Model file for the job. Use its own axes, mm. Coordinates: 2 decimals unless noted, no trailing zeros. Write each loop counter-clockwise with the first axis right and the second up, starting at its lowest first coordinate (ties: lowest second). Pieces come first, ordered by that corner, then holes. Notation, with made-up numbers: M 46.25,59 L 87.25,59 A12 ccw 87.25,82 Z; hole C 2.25,7.5 d1. An arc over 180 degrees is marked long. Use CSV: the item, a comma, the result in double quotes. Start each with the question number.
from build123d import *

# Parameters (mm, degrees)
SKETCH_1_R      = 1.6
SKETCH_1_R_2    = 1.65
EXTRUDE_1_DEPTH = 3.5


with BuildPart() as part:
    # 草图1 → 凸台-拉伸1 (new body)
    with BuildSketch(Plane(origin=(0, 0, 0), x_dir=(1, 0, 0), z_dir=(0, 1, 0))):
        with BuildLine():
            Line((8304.199636281, 3083.866766782), (8349.87122342, 3094.435360284))
            ThreePointArc((8349.87122342, 3094.435360284), (8352.100502408, 3095.843120102), (8352.969436472, 3098.332382262))
            Line((8352.969436472, 3098.332382262), (8352.969436472, 3114.411583007))
            ThreePointArc((8352.969436472, 3114.411583007), (8352.5356662, 3116.223213635), (8351.328433707, 3117.641928507))
            Line((8351.328433707, 3117.641928507), (8305.656846567, 3150.99413426))
            ThreePointArc((8305.656846567, 3150.99413426), (8302.988857908, 3151.75183644), (8300.469422208, 3150.592215885))
            Line((8300.469422208, 3150.592215885), (8292.469422208, 3142.592215885))
            ThreePointArc((8292.469422208, 3142.592215885), (8291.496370678, 3141.008280638), (8291.344362542, 3139.155560023))
            Line((8291.344362542, 3139.155560023), (8299.344362542, 3087.155560023))
            ThreePointArc((8299.344362542, 3087.155560023), (8301.054579793, 3084.452030652), (8304.199636281, 3083.866766782))
        make_face()
        with Locations(Location((8348.969436472, 3098.332382262, 0), (0, 0, 270))):
            Circle(SKETCH_1_R, mode=Mode.SUBTRACT)
        with Locations(Location((8348.969436472, 3114.411583007, 0), (0, 0, 270))):
            Circle(SKETCH_1_R, mode=Mode.SUBTRACT)
        with Locations(Location((8303.297849333, 3131.76378876, 0), (0, 0, 270))):
            Circle(SKETCH_1_R, mode=Mode.SUBTRACT)
        with Locations(Location((8303.297849333, 3087.76378876, 0), (0, 0, 270))):
            Circle(SKETCH_1_R, mode=Mode.SUBTRACT)
        with Locations(Location((8303.297849333, 3147.76378876, 0), (0, 0, 270))):
            Circle(SKETCH_1_R_2, mode=Mode.SUBTRACT)
        with Locations(Location((8295.297849333, 3139.76378876, 0), (0, 0, 270))):
            Circle(SKETCH_1_R_2, mode=Mode.SUBTRACT)
        with Locations(Location((8311.297849333, 3139.76378876, 0), (0, 0, 270))):
            Circle(SKETCH_1_R_2, mode=Mode.SUBTRACT)
    extrude(amount=EXTRUDE_1_DEPTH)


solid = part.part
1) Wall check: L1, parallel to X at y = 2.25, z = -3132.5; L2, parallel to Z at x = 8349, y = 0.3; L3, parallel to X at y = 1.5, z = -3118.5. Give the ranges that are in metal, low to high. Write a range as [from, to].
2) Band-saw the part on C-C on z = -3123. List the corners of the cut face in (x, y).
3) Two-plate mould, pull along Z, no slides. Class faces 1 (the face through (8296.69, 1.73, -3138.88)), 2 (the face through (8352.548, 1.726, -3116.2)), 3 (the face through (8322, 3.5, -3111)): pulls with the +Z half, pulls with the -Z half, needs draft (parallel to the pull), parting line crosses it, or undercut.
4) Band-saw the part on A-A on y = 1.9. List the corners of the cut face in (x, z), then the cut area to 3 significant figures.
5) Band-saw the part on B-B on x = 8326. List the corners of the cut face in (y, z), then the cut area to 3 significant figures.
Findings below:
1,L1,"x = [8292.37, 8301.88], [8304.72, 8330.98]"
1,L2,"z = [-3119.34, -3116.01], [-3112.81, -3099.93], [-3096.73, -3094.23]"
1,L3,"x = [8294.52, 8350.15]"
2,outline,"M 8293.83,0 L 8343.99,0 L 8343.99,3.5 L 8293.83,3.5 Z"
3,face 1,"undercut"
3,face 2,"pulls with the -Z half"
3,face 3,"needs draft"
4,outline,"M 8291.34,-3139.16 A4 ccw 8292.47,-3142.59 L 8300.47,-3150.59 A4 ccw 8305.66,-3150.99 L 8351.33,-3117.64 A4 ccw 8352.97,-3114.41 L 8352.97,-3098.33 A4 ccw 8349.87,-3094.44 L 8304.2,-3083.87 A4 ccw 8299.34,-3087.16 Z; hole C 8295.3,-3139.76 d3.3; hole C 8303.3,-3147.76 d3.3; hole C 8303.3,-3131.76 d3.2; hole C 8303.3,-3087.76 d3.2; hole C 8311.3,-3139.76 d3.3; hole C 8348.97,-3114.41 d3.2; hole C 8348.97,-3098.33 d3.2"
4,area,"2,700 mm2"
5,outline,"M 0,-3136.14 L 3.5,-3136.14 L 3.5,-3088.91 L 0,-3088.91 Z"
5,area,"165 mm2"
